Part model, mm, in its own coordinate system. Coordinates: 2 decimals unless noted, no trailing zeros. Order: outer loops, then holes, each group sorted by start corner. A loop starts at its lowest first (then second) coordinate and runs counter-clockwise, first axis right, second up.
1) Cut at A-A (x = -4). List the corners of the cut face in (y, z), and give its area (3 significant figures).
2) Pin check, flat tips, straight feed: pin 1 Ø1 at (y, z) = (-1, 1) entering from +X; pin 2 Ø4 at (x, z) = (28.5, 0) entering from +Y; pin 3 Ø1 at (x, y) = (-5.5, -2) entering from -Z. Stop position of each tip, or through.
3) Cut at C-C (x = 9). List the corners of the cut face in (y, z).
4) Cut at D-D (z = -15). List the corners of the cut face in (x, y).
5) Wall check: L1, parallel to Z at x = 28.5, y = -1.05; L2, parallel to X at y = -0.35, z = -7; L3, parallel to X at y = -2.1, z = 6.5. Give the ranges that are in metal, low to high.
6) Cut at B-B (y = -1.7). List the corners of the cut face in (x, z), and give its area (3 significant figures).
```python
from build123d import *

# Parameters (mm, degrees)
SKETCH1_R                = 10
BOSS_EXTRUDE1_DEPTH      = 3
M3_CLEARANCE_HOLE1_D     = 3.2
M3_CLEARANCE_HOLE1_DEPTH = 3


with BuildPart() as part:
    # Sketch1 → Boss-Extrude1 (new body)
    with BuildSketch(Plane(origin=(0, 0, 0), x_dir=(1, 0, 0), z_dir=(0, 1, 0))):
        with BuildLine():
            Line((-28.5, 3), (-23.314316453, 12.597327031))
            ThreePointArc((-23.314316453, 12.597327031), (0, 26.5), (23.314316453, 12.597327031))
            Line((23.314316453, 12.597327031), (28.5, 3))
            ThreePointArc((28.5, 3), (31.5, 0), (28.5, -3))
            Line((28.5, -3), (23.314316453, -12.597327031))
            ThreePointArc((23.314316453, -12.597327031), (0, -26.5), (-23.314316453, -12.597327031))
            Line((-23.314316453, -12.597327031), (-28.5, -3))
            ThreePointArc((-28.5, -3), (-31.5, 0), (-28.5, 3))
        make_face()
        Circle(SKETCH1_R, mode=Mode.SUBTRACT)
    extrude(amount=-BOSS_EXTRUDE1_DEPTH)

    # M3 Clearance Hole1
    with Locations(Plane(origin=(0, -3, 0), x_dir=(-1, 0, 0), z_dir=(0, -1, 0))):
        with Locations((-28.5, 0), (28.5, 0)):
            Hole(M3_CLEARANCE_HOLE1_D / 2, depth=M3_CLEARANCE_HOLE1_DEPTH)


solid = part.part
```
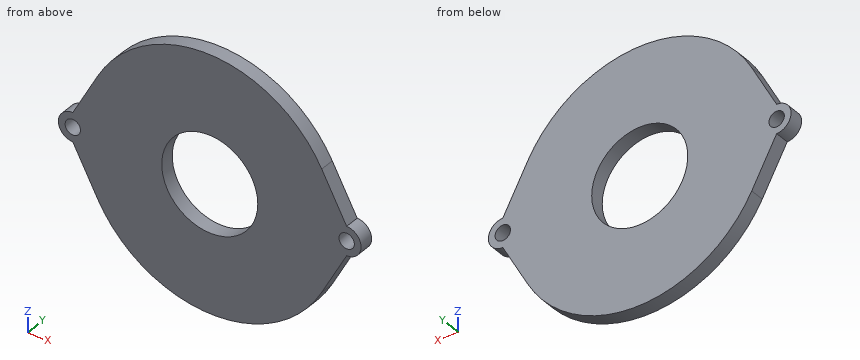
Geometry check:
1. outline: (-3, -26.2) - (0, -26.2) - (0, -9.17) - (-3, -9.17) - close; (-3, 9.17) - (0, 9.17) - (0, 26.2) - (-3, 26.2) - close
1. area: 102 mm2
2. pin 1: stops at x = 31.46
2. pin 2: stops at y = 0
2. pin 3: stops at z = -26.02
3. outline: (-3, -24.92) - (0, -24.92) - (0, -4.36) - (-3, -4.36) - close; (-3, 4.36) - (0, 4.36) - (0, 24.92) - (-3, 24.92) - close
4. outline: (-21.85, -3) - (21.85, -3) - (21.85, 0) - (-21.85, 0) - close
5. L1: z = -3 to -1.6, 1.6 to 3
5. L2: x = -26.34 to -7.14, 7.14 to 26.34
5. L3: x = -26.61 to -7.6, 7.6 to 26.61
6. outline: (-28.5, -3) - (-23.31, -12.6) arc R26.5 ccw to (23.31, -12.6) - (28.5, -3) arc R3 ccw to (28.5, 3) - (23.31, 12.6) arc R26.5 ccw to (-23.31, 12.6) - (-28.5, 3) arc R3 ccw to start; hole circle Ø3.2 at (-28.5, 0); hole circle Ø20 at (0, 0); hole circle Ø3.2 at (28.5, 0)
6. area: 1,960 mm2
